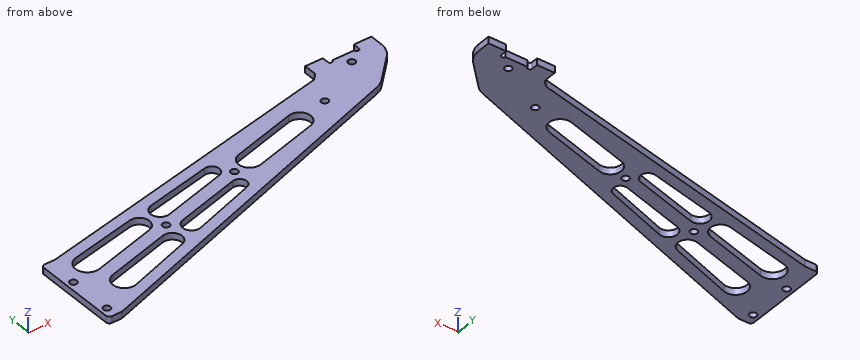
from build123d import *
from OCP.BRepFilletAPI import BRepFilletAPI_MakeChamfer

# Parameters (mm, degrees)
SKETCH_1_R          = 1.6
EXTRUDE_1_DEPTH     = 3
SKETCH_2_R          = 1.6
CUT_EXTRUDE_1_DEPTH = 3
CHAMFER_1_SIZE      = 2
CHAMFER_1_SIZE2     = 3.230198514
CHAMFER_1_SIZE2_2   = 2.634764865
SKETCH_3_R          = 1.6
CUT_EXTRUDE_2_DEPTH = 3
CUT_EXTRUDE_3_DEPTH = 3
FILLET_1_R          = 10
FILLET_2_R          = 1.5


with BuildPart() as part:
    # 草图1 → 凸台-拉伸1 (new body)
    with BuildSketch(Plane.XY):
        with BuildLine():
            Line((150, 32), (6.1, 0))
            Line((6.1, 0), (0, 0))
            Line((0, 0), (0, -40))
            Line((0, -40), (6.1, -40))
            Line((6.1, -40), (180, 20))
            Line((180, 20), (180, 40))
            Line((180, 40), (172, 40))
            Line((172, 40), (172, 37))
            ThreePointArc((172, 37), (171, 36), (170, 37))
            Line((170, 37), (160, 37))
            ThreePointArc((160, 37), (159, 36), (158, 37))
            Line((158, 37), (158, 40))
            Line((158, 40), (150, 40))
            Line((150, 40), (150, 32))
        make_face()
        with Locations((3.1, -35)):
            Circle(SKETCH_1_R, mode=Mode.SUBTRACT)
        with Locations((3.1, -15)):
            Circle(SKETCH_1_R, mode=Mode.SUBTRACT)
    extrude(amount=EXTRUDE_1_DEPTH)

    # 草图2 → 切除-拉伸1 (cut)
    with BuildSketch(Plane.XY.offset(3)):
        with Locations((165, 32)):
            Circle(SKETCH_2_R)
    extrude(amount=-CUT_EXTRUDE_1_DEPTH, mode=Mode.SUBTRACT)

    # 倒角1: one chamfer whose edges measure the first distance from different faces: ONE call of the kernel's chamfer builder (chamfer() names one face for all edges)
    chamfer_1_edges_1 = [part.edges().sort_by_distance(p)[0] for p in [
        (180, 20, 1.5),
    ]]
    chamfer_1_side_1 = [part.faces().sort_by_distance(p)[0] for p in [
        (93.05, -10, 1.5),
    ]]
    chamfer_1_edges_2 = [part.edges().sort_by_distance(p)[0] for p in [
        (150, 32, 1.5),
    ]]
    chamfer_1_side_2 = [part.faces().sort_by_distance(p)[0] for p in [
        (150, 36, 1.5),
    ]]
    chamfer_1 = BRepFilletAPI_MakeChamfer(part.part.solid().wrapped)
    for e in chamfer_1_edges_1:
        chamfer_1.Add(CHAMFER_1_SIZE, CHAMFER_1_SIZE2, e.wrapped, chamfer_1_side_1[0].wrapped)  # the first distance lies on this face
    for e in chamfer_1_edges_2:
        chamfer_1.Add(CHAMFER_1_SIZE, CHAMFER_1_SIZE2_2, e.wrapped, chamfer_1_side_2[0].wrapped)  # the first distance lies on this face
    add(Compound.cast(chamfer_1.Shape()), mode=Mode.REPLACE)

    # 草图3 → 切除-拉伸2 (cut)
    with BuildSketch(Plane.XY.offset(3)):
        with Locations((51.030979005, -7.253024477)):
            Circle(SKETCH_3_R)
        with Locations((90.458641741, 3.932653266)):
            Circle(SKETCH_3_R)
        with Locations((142.688604417, 18.75035968)):
            Circle(SKETCH_3_R)
        with BuildLine():
            Line((20.319493435, -29.80466571), (48.667912828, -20.023727449))
            ThreePointArc((48.667912828, -20.023727449), (51.382781252, -14.640684155), (46.077566644, -11.776707266))
            Line((46.077566644, -11.776707266), (17.22778338, -19.961427236))
            ThreePointArc((17.22778338, -19.961427236), (13.712756492, -26.472643184), (20.319493435, -29.80466571))
        make_face()
        with BuildLine():
            Line((97.96293832, 11.258954093), (126.823953345, 19.446860527))
            ThreePointArc((126.823953345, 19.446860527), (132.998773588, 16.001342428), (129.553255489, 9.826522185))
            Line((129.553255489, 9.826522185), (100.692240465, 1.638615751))
            ThreePointArc((100.692240465, 1.638615751), (94.517420222, 5.08413385), (97.96293832, 11.258954093))
        make_face()
        with BuildLine():
            Line((60.007280586, -16.111352144), (88.355699979, -6.330413883))
            ThreePointArc((88.355699979, -6.330413883), (90.334917033, -2.406020717), (86.467263213, -0.318099309))
            Line((86.467263213, -0.318099309), (57.617479949, -8.502819279))
            ThreePointArc((57.617479949, -8.502819279), (54.900467894, -13.53579706), (60.007280586, -16.111352144))
        make_face()
        with BuildLine():
            Line((15.590202093, -14.189224231), (44.439985357, -6.004504261))
            ThreePointArc((44.439985357, -6.004504261), (47.641256823, -0.456756962), (42.188030072, 2.902998549))
            Line((42.188030072, 2.902998549), (12.91477289, -3.60669033))
            ThreePointArc((12.91477289, -3.60669033), (8.806536259, -10.274778475), (15.590202093, -14.189224231))
        make_face()
        with BuildLine():
            Line((55.979898663, -2.730616274), (84.829681926, 5.454103696))
            ThreePointArc((84.829681926, 5.454103696), (87.188167139, 9.5413172), (83.170590126, 12.016562981))
            Line((83.170590126, 12.016562981), (53.897332945, 5.506874101))
            ThreePointArc((53.897332945, 5.506874101), (50.699463699, 0.316405313), (55.979898663, -2.730616274))
        make_face()
    extrude(amount=-CUT_EXTRUDE_2_DEPTH, mode=Mode.SUBTRACT)

    # 草图4 → 切除-拉伸3 (cut)
    with BuildSketch(Plane.XY.offset(3)):
        Polygon((180, 30), (165, 14.824611846), (178.109369602, 19.347683589), (180, 23.230198514), align=None)
    extrude(amount=-CUT_EXTRUDE_3_DEPTH, mode=Mode.SUBTRACT)

    # 圆角1
    fillet_1_edges = [part.edges().sort_by_distance(p)[0] for p in [
        (180, 30, 1.5),
        (165, 14.824611846, 1.5),
    ]]
    fillet(fillet_1_edges, radius=FILLET_1_R)

    # 圆角2
    fillet_2_edges = [part.edges().sort_by_distance(p)[0] for p in [
        (6.1, -40, 1.5),
        (0, -40, 1.5),
        (0, 0, 1.5),
        (6.1, 0, 1.5),
        (147.428060769, 31.428060769, 1.5),
        (150, 34, 1.5),
    ]]
    fillet(fillet_2_edges, radius=FILLET_2_R)


solid = part.part
Could you check a few things on this model? Use its own coordinates, in mm. Round coordinates to 2 decimals unless told otherwise and drop trailing zeros. Write each loop counter-clockwise with the first axis right and the second up, starting at its lowest first coordinate (ties: lowest second). Pieces come first, ordered by that corner, then holes. Notation, with made-up numbers: (84, -17.75) - (114, -17.75) arc R11 ccw to (114, -5.75) - close; hole circle Ø9 at (-27.5, 76.25). An arc over 180 degrees is marked (long way). Put each result on its own line as item: value. Start each with the question number.
(1) I want a section at A-A, the plane x = 3.1. Please give me the cut outline in (y, z).
(2) Will these pins go through, and if not, where does the flat tip stop? pin 1 (1.5 mm diameter, centred on y = 38, z = 1, fed in from -X); pin 2 (1.5 mm diameter, centred on x = 66, z = 0.5, fed in from -Y); pin 3 (2.5 mm diameter, centred on x = 142.69, y = 18.75, fed in from -Z); pin 4 (1 mm diameter, centred on x = 31.5, z = 2, fed in from +Y).
(3) I need wall thicknesses on probe 1 along Y at (x, z) = (3.1, 1.1); probe 2 along Y at (x, z) = (89, 0.65); probe 3 along Y at (x, z) = (113.5, 1.5). Which ranges of each line are inside material? Lowest first, please.
(4) I want a section at B-B, the plane y = -35. Please give me the cut outline in (x, z).
(5) I want a section at D-D, the plane x = 32.5. Please give me the cut outline in (y, z).
(6) I want a section at C-C, the plane x = 106. Please give me the cut outline in (y, z).
Here are the results:
1. outline: (-40, 0) - (-36.6, 0) - (-36.6, 3) - (-40, 3) - close; (-33.4, 0) - (-16.6, 0) - (-16.6, 3) - (-33.4, 3) - close; (-13.4, 0) - (0, 0) - (0, 3) - (-13.4, 3) - close
2. pin 1: stops at x = 150
2. pin 2: stops at y = -19.59
2. pin 3: passes through
2. pin 4: stops at y = 5.76
3. probe 1: y = -40 to -36.6, -33.4 to -16.6, -13.4 to 0
3. probe 2: y = -11.4 to -6.02, -0.68 to 3.28, 4.59 to 18.44
3. probe 3: y = -2.94 to 5.27, 15.67 to 23.88
4. outline: (0, 0) - (1.5, 0) - (1.5, 3) - (0, 3) - close; (4.7, 0) - (20.59, 0) - (20.59, 3) - (4.7, 3) - close
5. outline: (-30.89, 0) - (-25.6, 0) - (-25.6, 3) - (-30.89, 3) - close; (-15.63, 0) - (-9.39, 0) - (-9.39, 3) - (-15.63, 3) - close; (0.75, 0) - (5.87, 0) - (5.87, 3) - (0.75, 3) - close
6. outline: (-5.53, 0) - (3.14, 0) - (3.14, 3) - (-5.53, 3) - close; (13.54, 0) - (22.22, 0) - (22.22, 3) - (13.54, 3) - close
